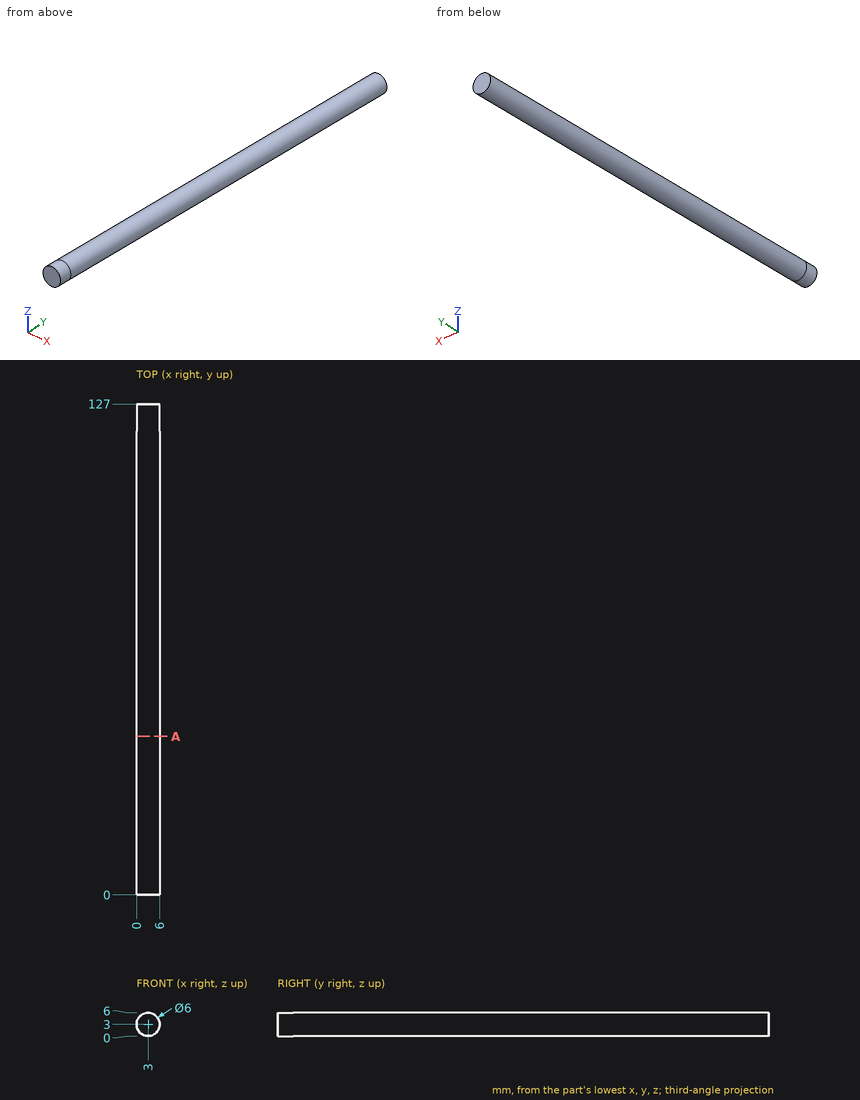
Check sheet for the drawn part. Datum: minimum x, y, z corner. Units: mm. Coordinates: 2 decimals unless noted, no trailing zeros. Loops run counter-clockwise (first coordinate to the right, second up) from the corner with the lowest first, then second, coordinate; pieces in that order, holes last. Notation, with made-up numbers: (2.25, 55.25) -> (14.25, 55.25) arc R19 cw to (14.25, 79.25) -> close; hole circle Ø8 at (37.25, -7). An arc over 180 degrees is marked (long way). Answer in a Markdown table with one row per item.
1) Depth check by flat-ended pin: P1, Ø2, axis at x = 1.5, y = 20, coming from the -Z side; P2, Ø1, axis at x = 4.5, y = 27.5, coming from the -Z side. Enter the tip coordinate at first touch or a pass-through.
The answers:
| item | result |
|---|---|
| P1 | stops at z = 0.04 |
| P2 | stops at z = 0.17 |
2) Scan lines: line 1 along X through (y, z) = (119, 4.45); line 2 along X through (y, z) = (58.5, 2.3); line 3 along Z through (x, y) = (4.05, 11). Record each from-to range of solid material in increasing order. Write a range as from..to.
The answers:
| item | result |
|---|---|
| line 1 | x = 0.37..5.63 |
| line 2 | x = 0.08..5.92 |
| line 3 | z = 0.19..5.81 |
3) Section check A-A (y = 41). Record the cut outline in (x, z).
The answers:
| item | result |
|---|---|
| outline | circle Ø6 at (3, 3) |
